Autodesk Fusion 360 part; units mm, degrees
sketch "Sketch1" plane through (0, 0, 0) normal (0, 0, 1) x (1, 0, 0)
  circle A0 centre (0, 0) radius 35
  circle A1 centre (0, 0) radius 25
  circle A2 centre (0, 0) radius 28 construction
  circle A3 centre (0, 0) radius 32 construction
  dimension "d1" = 70
  dimension "d2" = 50
  dimension "d6" = 56
  dimension "d15" = 4
extrude "Extrude1" add sketch "Sketch1" along normal blind 3
sketch "Sketch2" plane through (0, 0, 0) normal (0, 0, -1) x (1, 0, 0)
  circle A0 centre (0, 0) radius 25
  circle A1 centre (0, 0) radius 35
  circle A2 centre (0, 0) radius 28 construction
  arc A3 (4.8393, 26.6644) -> (-4.8393, 26.6644) centre (0, 0) ccw
  arc A4 (4.8393, 26.6644) -> (5.1607, 28.4355) centre (5, 27.55) ccw
  arc A5 (5.1607, 28.4355) -> (-5.1607, 28.4355) centre (0, 0) ccw
  arc A6 (-5.1607, 28.4355) -> (-4.8393, 26.6644) centre (-5, 27.55) ccw
  arc A7 (5, 27.55) -> (-5, 27.55) centre (0, 0) ccw construction
  line L0 (-5, 27.55) -> (5, 27.55) construction
  line L1 (0, 0) -> (0, 55.0999) construction
  dimension "d5" = 56
  dimension "d7" = 0.9
  dimension "d14" = 10
extrude "Extrude2" add sketch "Sketch2" along normal blind 2.5 contours A3 A4 A5 A6
pattern_circular "C-Pattern1" count 4 over 360 about axis through (0, 0, 0) along (0, 0, -1) of "Extrude2"
CAD build for the part. Positions are in the model's coordinates, mm. A direction names the side the tool comes from. Give positions to 0.01 mm unless a question says otherwise; leave off trailing zeros. Order: outer loops, then holes, each group sorted by start corner. A loop starts at its lowest first (then second) coordinate and runs counter-clockwise, first axis right, second up. Notation, with made-up numbers: M 65,17 L 91,17 A20 ccw 91,48 Z; hole C -20.5,-17.75 d2. An arc over 180 degrees is marked long. Put each result on its own line as item: value. Start each with the question number.
(1) Saw through at D-D, the plane x = 19.5. Write the cut outline in (y, z), then the cut area to 3 significant figures.
(2) Flat gauge pins, fed straight in: pin 1 Ø1.5 at (y, z) = (-21, 2) entering from -X; pin 2 Ø3 at (y, z) = (8, -1) entering from -X; pin 3 Ø3 at (y, z) = (2.5, 2) entering from -X. Where does each tip first touch, or does it go through?
(3) Which spindle directions (+Z, -Z, +X, -X, +Y, -Y) get a long thin tool onto all of the face, cutting with end or side? Do faces 1 (the cylindrical face through (-0.1, -27.1, -1.2)), 2 (the cylindrical face through (-0.1, -28.9, -1.2)), 3 (the cylindrical face through (-28.9, 0.1, -1.2)). Say none if no direction does.
(4) Saw through at A-A, the plane y = 0. Write the cut outline in (x, z), then the cut area to 3 significant figures.
(5) Drill centre lines: line 1 along Y through (x, z) = (0, 2.4); line 2 along Z through (x, y) = (25, 2); line 3 along Y through (x, z) = (6, 2.4). Where is each one in solid material? Low to high.
(6) Mould opens along X. For faces 4 (the flat face through (0, -28, -2.5)), 5 (the cylindrical face through (-28, 21, 1)), 6 (the cylindrical face through (0.1, 27.1, -1.2)) say: +X half, -X half, draft (parallel to the pull), parting line (faces both ways), or undercut.
(7) Saw through at B-B, the plane z = -1.25. Write the cut outline in (x, y), then the cut area to 3 significant figures.
Check result:
1. outline: M -29.06,0 L -15.64,0 L -15.64,3 L -29.06,3 Z; M 15.64,0 L 29.06,0 L 29.06,3 L 15.64,3 Z
1. area: 80.5 mm2
2. pin 1: stops at x = -28.55
2. pin 2: stops at x = -34.32
2. pin 3: stops at x = -34.99
3. face 1: -Z
3. face 2: -Z, -Y
3. face 3: -Z, -X
4. outline: M -35,0 L -28.9,0 L -28.9,-2.5 L -27.1,-2.5 L -27.1,0 L -25,0 L -25,3 L -35,3 Z; M 25,0 L 27.1,0 L 27.1,-2.5 L 28.9,-2.5 L 28.9,0 L 35,0 L 35,3 L 25,3 Z
4. area: 69.0 mm2
5. line 1: y = -35 to -25, 25 to 35
5. line 2: z = 0 to 3
5. line 3: y = -34.48 to -24.27, 24.27 to 34.48
6. face 4: draft
6. face 5: parting line
6. face 6: undercut
7. outline: M -28.44,-5.16 A0.9 ccw -26.66,-4.84 A27.1 cw -26.66,4.84 A0.9 ccw -28.44,5.16 A28.9 ccw Z; M -5.16,-28.44 A28.9 ccw 5.16,-28.44 A0.9 ccw 4.84,-26.66 A27.1 cw -4.84,-26.66 A0.9 ccw Z; M -5.16,28.44 A0.9 ccw -4.84,26.66 A27.1 cw 4.84,26.66 A0.9 ccw 5.16,28.44 A28.9 ccw Z; M 26.66,-4.84 A0.9 ccw 28.44,-5.16 A28.9 ccw 28.44,5.16 A0.9 ccw 26.66,4.84 A27.1 cw Z
7. area: 82.6 mm2
